```python
from build123d import *

# Parameters (mm, degrees)
SKETCH_W     = 15
SKETCH_H     = 50
PAD_DEPTH    = 5
PAD001_DEPTH = 15


with BuildPart() as part:
    # Sketch → Pad (new body)
    with BuildSketch(Plane.XY):
        Rectangle(SKETCH_W, SKETCH_H)
    extrude(amount=PAD_DEPTH)

    # Sketch001 (on Face3 of Pad) → Pad001 (join)
    with BuildSketch(Plane.YZ.offset(7.5)):
        Polygon((-23.75, 5), (-23.5, 6), (-21.5, 6), (-21.25, 5), align=None)
        Polygon((-18.75, 5), (-18.5, 6), (-16.5, 6), (-16.25, 5), align=None)
        Polygon((-13.75, 5), (-13.5, 6), (-11.5, 6), (-11.25, 5), align=None)
        Polygon((-8.75, 5), (-8.5, 6), (-6.5, 6), (-6.25, 5), align=None)
        Polygon((-3.75, 5), (-3.5, 6), (-1.5, 6), (-1.25, 5), align=None)
        Polygon((1.25, 5), (1.5, 6), (3.5, 6), (3.75, 5), align=None)
        Polygon((6.25, 5), (6.5, 6), (8.5, 6), (8.75, 5), align=None)
        Polygon((11.25, 5), (11.5, 6), (13.5, 6), (13.75, 5), align=None)
        Polygon((16.25, 5), (16.5, 6), (18.5, 6), (18.75, 5), align=None)
        Polygon((21.25, 5), (21.5, 6), (23.5, 6), (23.75, 5), align=None)
    extrude(amount=-PAD001_DEPTH)


solid = part.part
```
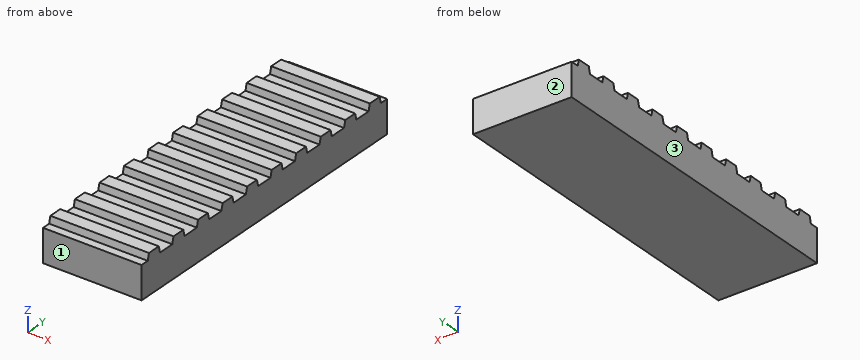
The model under review builds one solid part; all positions refer to its coordinate system, in mm. Face numbers are marked on the shaded views. Round coordinates to 2 decimals unless told otherwise and drop trailing zeros. Loops run counter-clockwise (first coordinate to the right, second up) from the corner with the lowest first, then second, coordinate; pieces in that order, holes last. Notation, with made-up numbers: (68.25, -26.75) - (87.25, -26.75) arc R13 cw to (87.25, -8.75) - close; hole circle Ø10 at (28.5, 27.25). An arc over 180 degrees is marked (long way). Use a Markdown table: item, result. Add a question column.
Q1. Insertion check: pin 1 Ø1.2 at (x, y) = (-2.5, -10.5) entering from +Z. The pin has a flat end and moves straight along its axis. Give the tip position at first contact, or say it passes through.
Q2. For probe 1 along Z at (x, y) = (3.75, -10), list the stretches that pass through material, from the lowest coordinate up.
Q3. Add section A-A (y = 15.5). State the section outline as (x, z) points, plus the area to 3 significant figures.
Q4. The part is to be moulded in two halves that separate along Y. For the marked faces 1, 2 and 3, say which applies: pulls with the +Y half, pulls with the -Y half, needs draft (parallel to the pull), parting line crosses it, or undercut.
Worked answers:
| question | item | result |
|---|---|---|
| 1 | pin 1 | z = 5 |
| 2 | probe 1 | 0 to 5 |
| 3 | outline | (-7.5, 0) - (7.5, 0) - (7.5, 5) - (-7.5, 5) - close |
| 3 | area | 75.0 mm² |
| 4 | face 1 | pulls with the -Y half |
| 4 | face 2 | pulls with the +Y half |
| 4 | face 3 | needs draft |
